from build123d import *

# Parameters (mm, degrees)
SKETCH1_R               = 14
BOSS_EXTRUDE1_DEPTH     = 550
SKETCH2_R               = 8
CUT_EXTRUDE1_DEPTH      = 15
CUT_EXTRUDE1_DEPTH_BACK = 15
CHAMFER1_SIZE           = 3


with BuildPart() as part:
    # Sketch1 → Boss-Extrude1 (new body)
    with BuildSketch(Plane(origin=(0, 0, 0), x_dir=(1, 0, 0), z_dir=(0, 1, 0))):
        Circle(SKETCH1_R)
    extrude(amount=BOSS_EXTRUDE1_DEPTH)

    # Sketch2 → Cut-Extrude1 (cut, two sides)
    with BuildSketch(Plane.XY) as cut_extrude1_sk:
        with Locations((0, 530)):
            Circle(SKETCH2_R)
    extrude(amount=CUT_EXTRUDE1_DEPTH, mode=Mode.SUBTRACT)
    extrude(cut_extrude1_sk.sketch, amount=-CUT_EXTRUDE1_DEPTH_BACK, mode=Mode.SUBTRACT)

    # Chamfer1
    chamfer1_edges = [part.edges().sort_by_distance(p)[0] for p in [
        (-14, 0, 0),
        (-14, 550, 0),
    ]]
    chamfer(chamfer1_edges, length=CHAMFER1_SIZE)


solid = part.part
Verification items for the finished model (mm, model axes). Give positions to 0.01 mm unless a question says otherwise; leave off trailing zeros. Write each loop counter-clockwise with the first axis right and the second up, starting at its lowest first coordinate (ties: lowest second). Pieces come first, ordered by that corner, then holes. Notation, with made-up numbers: M 52,19.25 L 77,19.25 A18 ccw 77,51.25 Z; hole C 39.25,58.5 d3. An arc over 180 degrees is marked long. Use CSV: the item, a comma, the result in double quotes.
1) Release check for a two-part mould opening along Y. For faces 1 (the face through (-8.845, 549.854, 6.782)), 2 (the face through (-5.9, 535.4, 0.2)), 3 (the face through (0, 0, 0)) record: released by +Y, released by -Y, zero draft, split by the parting line, or undercut.
Final values:
face 1,"released by +Y"
face 2,"undercut"
face 3,"released by -Y"
2) Material ranges on line 1 along X through (y, z) = (530, 1); line 2 along Y through (x, z) = (0, 0.75); line 3 along Y through (x, z) = (4.5, 4), recorded low to high.
Final values:
line 1,"-13.96 to -8, 8 to 13.96"
line 2,"0 to 522, 538 to 550"
line 3,"0 to 523.39, 536.61 to 550"
3) Cross-section at A-A (x = 0). Enter the section's corners in (y, z), plus the area to 3 significant figures.
Final values:
outline,"M 0,-11 L 3,-14 L 522,-14 L 522,14 L 3,14 L 0,11 Z; M 538,-14 L 547,-14 L 550,-11 L 550,11 L 547,14 L 538,14 Z"
area,"14,900 mm²"
4) Go/stop test with flat-tipped pins: pin 1 Ø4 at (x, y) = (-5, 449) entering from +Z; pin 2 Ø10 at (y, z) = (468.5, -6.5) entering from +X; pin 3 Ø8 at (y, z) = (404, -8) entering from -X. Record where each tip stops, or that it passes through.
Final values:
pin 1,"z = 13.67"
pin 2,"x = 13.92"
pin 3,"x = -13.42"
5) Cross-section at B-B (y = 530). Enter the section's corners in (x, z), plus the area to 3 significant figures.
Final values:
outline,"M -8,-11.49 L -8,11.49 A14 ccw Z; M 8,-11.49 A14 ccw 8,11.49 Z"
area,"193 mm²"
